```python
from build123d import *

# Parameters (mm, degrees)
F1_DEPTH = 241.3
F2_R     = 6.35
F3_DEPTH = 50.8
F4_R     = 6.35
F5_DEPTH = 25.4


with BuildPart() as f1:
    # F0 (on Front) → F1 (new body)
    with BuildSketch(Plane.XZ):
        Polygon((-10.16, 0), (0, 0), (91.44, 0), (91.44, 10.16), (0, 10.16), (0, 101.6), (-10.16, 101.6), (-10.16, 10.16), align=None)
    extrude(amount=F1_DEPTH)

    # F2 (on face) → F3 (cut)
    with BuildSketch(Plane.XY.offset(10.16)):
        with Locations((27.94, -25.4)):
            Circle(F2_R)
        with Locations((66.04, -63.5)):
            Circle(F2_R)
        with Locations((66.04, -177.8)):
            Circle(F2_R)
        with Locations((27.94, -215.9)):
            Circle(F2_R)
    extrude(amount=-F3_DEPTH, mode=Mode.SUBTRACT)

    # F4 (on face) → F5 (cut)
    with BuildSketch(Plane.YZ):
        with Locations((-177.8, 60.96)):
            Circle(F4_R)
        with Locations((-63.5, 60.96)):
            Circle(F4_R)
    extrude(amount=-F5_DEPTH, mode=Mode.SUBTRACT)


solid = f1.part
```
Check sheet for the modelled part. Datum: model origin and axes. Units: mm. A direction names the side the tool comes from. Coordinates: 2 decimals unless noted, no trailing zeros. Order: outer loops, then holes, each group sorted by start corner. A loop starts at its lowest first (then second) coordinate and runs counter-clockwise, first axis right, second up. Notation, with made-up numbers: (73.5, -33) -> (130.5, -33) arc R10 ccw to (130.5, -21) -> close; hole circle Ø4 at (42.5, 13.25). An arc over 180 degrees is marked (long way). Write item = value, one per line. Start each with the question number.
1) Access from +Z, -Z, +X, -X, +Y, -Y to the whole of each face (thin tool, end or side, straight path). Record for faces 1 (the flat face through (0, -119, 55)), 2 (the flat face through (18, -241.3, 10)).
2) Cross-section at A-A (z = 60.96). Enter the section's corners in (x, y).
3) Cross-section at C-C (x = 27.94). Enter the section's corners in (y, z).
4) Go/stop test with flat-tipped pins: P1, Ø20.5, axis at x = 66.04, y = -63.5, coming from the +Z side; P2, Ø11.5, axis at y = -177.8, z = 60.96, coming from the -X side. Record where each tip stops, or that it passes through.
5) Cross-section at B-B (y = -215.9). Enter the section's corners in (x, z), then the cut area to 3 significant figures.
6) Mould release check, pull along Z, two halves, no side actions. Record for faces 3 (the flat face through (46, -119, 10.16)), 4 (the cylindrical face through (-5.009, -184.144, 61.239)), 5 (the flat face through (40, -119, 0)): +Z half, -Z half, draft (parallel to the pull), parting line (faces both ways), or undercut.
7) Material ranges on L1, parallel to Y at x = 27.94, z = 7.5; L2, parallel to Y at x = 66.04, z = 6; L3, parallel to Z at x = -3.75, y = -63.5, recorded low to high.
8) Cross-section at D-D (y = -177.8). Enter the section's corners in (x, z).
Ans:
q1.face_1 = +Z, +X, +Y, -Y
q1.face_2 = +Z, -Z, +X, -X, -Y
q2.outline = (-10.16, -241.3) -> (0, -241.3) -> (0, -184.15) -> (-10.16, -184.15) -> close; (-10.16, -171.45) -> (0, -171.45) -> (0, -69.85) -> (-10.16, -69.85) -> close; (-10.16, -57.15) -> (0, -57.15) -> (0, 0) -> (-10.16, 0) -> close
q3.outline = (-241.3, 0) -> (-222.25, 0) -> (-222.25, 10.16) -> (-241.3, 10.16) -> close; (-209.55, 0) -> (-31.75, 0) -> (-31.75, 10.16) -> (-209.55, 10.16) -> close; (-19.05, 0) -> (0, 0) -> (0, 10.16) -> (-19.05, 10.16) -> close
q4.P1 = 10.16
q4.P2 = through
q5.outline = (-10.16, 0) -> (21.59, 0) -> (21.59, 10.16) -> (0, 10.16) -> (0, 101.6) -> (-10.16, 101.6) -> close; (34.29, 0) -> (91.44, 0) -> (91.44, 10.16) -> (34.29, 10.16) -> close
q5.area = 1,830 mm²
q6.face_3 = +Z half
q6.face_4 = undercut
q6.face_5 = -Z half
q7.L1 = -241.3 to -222.25, -209.55 to -31.75, -19.05 to 0
q7.L2 = -241.3 to -184.15, -171.45 to -69.85, -57.15 to 0
q7.L3 = 0 to 54.61, 67.31 to 101.6
q8.outline = (-10.16, 0) -> (59.69, 0) -> (59.69, 10.16) -> (0, 10.16) -> (0, 54.61) -> (-10.16, 54.61) -> close; (-10.16, 67.31) -> (0, 67.31) -> (0, 101.6) -> (-10.16, 101.6) -> close; (72.39, 0) -> (91.44, 0) -> (91.44, 10.16) -> (72.39, 10.16) -> close
